Design review of the part built by this model. Coordinates are the model's own, in mm. Face numbers are marked on the shaded views. A direction names the side the tool comes from. Coordinates: 2 decimals unless noted, no trailing zeros. Order: outer loops, then holes, each group sorted by start corner. A loop starts at its lowest first (then second) coordinate and runs counter-clockwise, first axis right, second up. Notation, with made-up numbers: (3, -12) - (28, -12) arc R32 cw to (28, 26) - close; hole circle Ø6 at (11.25, 84). An arc over 180 degrees is marked (long way). Write each question's results on one line, items separated by ' | '. Start each with the question number.
```python
from build123d import *

# Parameters (mm, degrees)
DODANIE_WYCI_GNI_CIE1_DEPTH = 12
SZKIC2_R                    = 2.1
WYTNIJ_WYCI_GNI_CIE1_DEPTH  = 10
WYTNIJ_WYCI_GNI_CIE2_DEPTH  = 42
WYTNIJ_WYCI_GNI_CIE3_REACH  = 51.366
SZKIC4_R                    = 2.1
WYTNIJ_WYCI_GNI_CIE4_DEPTH  = 6


with BuildPart() as part:
    # Szkic1 → Dodanie-wyciągnięcie1 (new body)
    with BuildSketch(Plane.XY):
        with BuildLine():
            Line((-23, 0), (23, 0))
            Line((23, 0), (23, 14))
            Line((23, 14), (18, 19))
            Line((18, 19), (18, 51))
            Line((18, 51), (23, 56))
            Line((23, 56), (23, 70))
            Line((23, 70), (7, 70))
            Line((7, 70), (7, 35))
            ThreePointArc((7, 35), (0, 28), (-7, 35))
            Line((-7, 35), (-7, 70))
            Line((-7, 70), (-23, 70))
            Line((-23, 70), (-23, 56))
            Line((-23, 56), (-18, 51))
            Line((-18, 51), (-18, 19))
            Line((-18, 19), (-23, 14))
            Line((-23, 14), (-23, 0))
        make_face()
    extrude(amount=DODANIE_WYCI_GNI_CIE1_DEPTH)

    # Szkic2 → Wytnij-wyciągnięcie1 (cut)
    with BuildSketch(Plane(origin=(0, 70, 0), x_dir=(1, 0, 0), z_dir=(0, 1, 0))):
        with Locations(Location((-19, -6, 0), (0, 0, 270))):
            Circle(SZKIC2_R)
        with Locations(Location((19, -6, 0), (0, 0, 270))):
            Circle(SZKIC2_R)
    wytnij_wyci_gni_cie1 = extrude(amount=-WYTNIJ_WYCI_GNI_CIE1_DEPTH, mode=Mode.SUBTRACT)

    # Lustro1: Wytnij-wyciągnięcie1 across plane
    add(wytnij_wyci_gni_cie1.mirror(Plane(origin=(0, 35, 0), x_dir=(0, 0, 1), z_dir=(0, -1, 0))), mode=Mode.SUBTRACT)

    # Szkic3 → Wytnij-wyciągnięcie2 (cut)
    with BuildSketch(Plane(origin=(0, 70, 0), x_dir=(-1, 0, 0), z_dir=(0, -1, 0))):
        Polygon((12.6, -2), (-12.6, -2), (-15, -4.4), (-15, -7.6), (-12.6, -10), (12.6, -10), (15, -7.6), (15, -4.4), align=None)
    extrude(amount=WYTNIJ_WYCI_GNI_CIE2_DEPTH, mode=Mode.SUBTRACT)

    # Szkic4 → Wytnij-wyciągnięcie3 (cut, up to next)
    with BuildSketch(Plane(origin=(0, 28, 0), x_dir=(1, 0, 0), z_dir=(0, 1, 0)), mode=Mode.PRIVATE) as wytnij_wyci_gni_cie3_sk1:
        with Locations(Location((11, -6, 0), (0, 0, 270))):
            Circle(SZKIC4_R)
    wytnij_wyci_gni_cie3_tool1 = extrude(wytnij_wyci_gni_cie3_sk1.sketch, amount=-WYTNIJ_WYCI_GNI_CIE3_REACH, mode=Mode.PRIVATE) & part.part
    # Szkic4 → Wytnij-wyciągnięcie3 (cut, up to next)
    with BuildSketch(Plane(origin=(0, 28, 0), x_dir=(1, 0, 0), z_dir=(0, 1, 0)), mode=Mode.PRIVATE) as wytnij_wyci_gni_cie3_sk2:
        with Locations(Location((-11, -6, 0), (0, 0, 270))):
            Circle(SZKIC4_R)
    wytnij_wyci_gni_cie3_tool2 = extrude(wytnij_wyci_gni_cie3_sk2.sketch, amount=-WYTNIJ_WYCI_GNI_CIE3_REACH, mode=Mode.PRIVATE) & part.part
    add(wytnij_wyci_gni_cie3_tool1.solids().sort_by_distance((11, 28, 6))[0], mode=Mode.SUBTRACT)
    add(wytnij_wyci_gni_cie3_tool2.solids().sort_by_distance((-11, 28, 6))[0], mode=Mode.SUBTRACT)

    # Szkic5 → Wytnij-wyciągnięcie4 (cut)
    with BuildSketch(Plane.XZ):
        Polygon((11, 1.727608008), (14.7, 3.863804004), (14.7, 8.136195996), (11, 10.272391992), (7.3, 8.136195996), (7.3, 3.863804004), align=None)
        Polygon((-7.3, 3.863804004), (-11, 1.727608008), (-14.7, 3.863804004), (-14.7, 8.136195996), (-11, 10.272391992), (-7.3, 8.136195996), align=None)
    extrude(amount=-WYTNIJ_WYCI_GNI_CIE4_DEPTH, mode=Mode.SUBTRACT)


solid = part.part
```
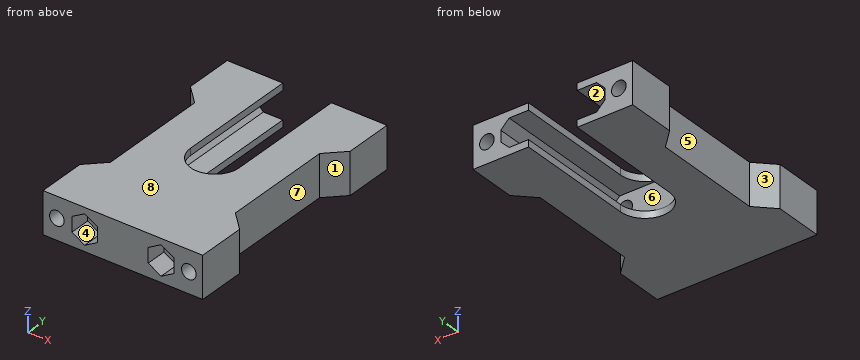
(1) Take a section at D-D (z = 6). State how many separate pieces and enclosed holes the cut face has, plus the area to 3 significant figures.
(2) Clearance check with flat-ended pins moving along their axes: pin 1 (6 mm diameter, centred on y = 39, z = 7, fed in from -X); pin 2 (4 mm diameter, centred on x = 6.5, z = 5.5, fed in from +Y); pin 3 (2.5 mm diameter, centred on y = 49, z = 6, fed in from +X). State where each tip first meets the part, or that it passes through.
(3) Take a section at B-B (x = 19). State the section outline as (y, z) points, plus the area to 3 significant figures.
(4) Tool access review of the marked faces 1, 2, 3 and 4: name each direction out of +Z, -Z, +X, -X, +Y, -Y from which nothing blocks a thin tool from reaching the whole face with its end or side.
(5) Mouldability with a two-part tool opening along X and no side actions: class the marked faces 5, 6, 7 and 8 as +X half, -X half, draft (parallel to the pull), parting line (faces both ways), or undercut.
(6) Take a section at C-C (y = 44). State the section outline as (x, z) points.
(7) To check wall thickness, follow line 1 along X through (y, z) = (12, 6); line 2 along X through (y, z) = (3.75, 6); line 3 along X through (y, z) = (66.5, 6). State the ranges of each line that lie inside material, in increasing order. Write a range as [from, to].
(8) Take a section at A-A (y = 11). State the section outline as (x, z) points, plus the area to 3 significant figures.
Worked out:
1) separate pieces: 3 | enclosed holes: 0 | area: 1,150 mm^2
2) pin 1: x = -18 | pin 2: y = 28 | pin 3: x = 18
3) outline: (0, 0) - (18, 0) - (18, 12) - (0, 12) - (0, 8.1) - (10, 8.1) - (10, 3.9) - (0, 3.9) - close; (52, 0) - (70, 0) - (70, 3.9) - (60, 3.9) - (60, 8.1) - (70, 8.1) - (70, 12) - (52, 12) - close | area: 348 mm^2
4) face 1: +Z, -Z, +X | face 2: +Y | face 3: +Z, -Z, -X | face 4: -Y
5) face 5: -X half | face 6: undercut | face 7: +X half | face 8: draft
6) outline: (-18, 0) - (-7, 0) - (-7, 2) - (-12.6, 2) - (-15, 4.4) - (-15, 7.6) - (-12.6, 10) - (-7, 10) - (-7, 12) - (-18, 12) - close; (7, 0) - (18, 0) - (18, 12) - (7, 12) - (7, 10) - (12.6, 10) - (15, 7.6) - (15, 4.4) - (12.6, 2) - (7, 2) - close
7) line 1: [-23, -13.1], [-8.9, 8.9], [13.1, 23] | line 2: [-23, -21.1], [-16.9, -14.7], [-7.3, 7.3], [14.7, 16.9], [21.1, 23] | line 3: [-23, -21.1], [-16.9, -15], [15, 16.9], [21.1, 23]
8) outline: (-23, 0) - (23, 0) - (23, 12) - (-23, 12) - close; hole circle Ø4.2 at (-11, 6); hole circle Ø4.2 at (11, 6) | area: 524 mm^2
